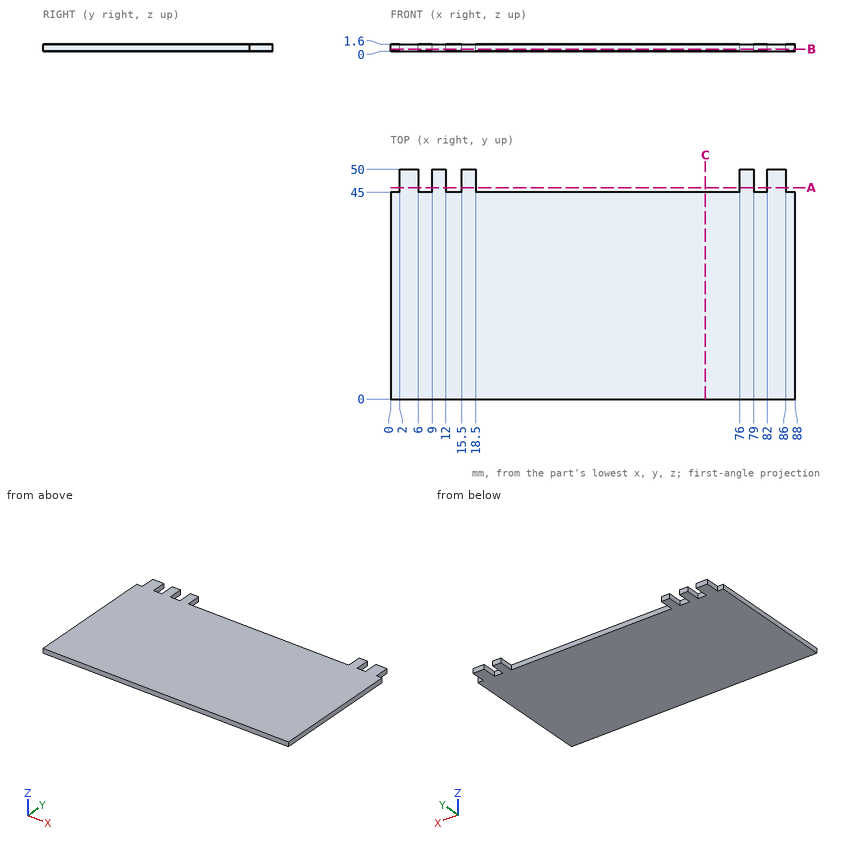
Source: three-view drawing plus pictorial views. Frame: mm from the lowest corner of the part. Give positions to 0.01 mm unless a question says otherwise; leave off trailing zeros. Write each loop counter-clockwise with the first axis right and the second up, starting at its lowest first coordinate (ties: lowest second). Pieces come first, ordered by that corner, then holes. Notation, with made-up numbers: M -5,68 L 1,68 A14 cw 1,72 Z; hole C -36,-17.5 d3. An arc over 180 degrees is marked long. Use one line per item in the form item = value.
1. Ray query, L1, parallel to X at y = 47.5, z = 1.15; L2, parallel to Y at x = 36, z = 1.35. Return the intervals inside material, ascending.
Outcome:
L1 = 2 to 6, 9 to 12, 15.5 to 18.5, 76 to 79, 82 to 86
L2 = 0 to 45
2. First-contact query: P1, Ø0.8, axis at x = 45.5, z = 1, coming from the +Y side; P2, Ø0.8, axis at y = 47.5, z = 1, coming from the -X side; P3, Ø0.5, axis at y = 47.5, z = 1, coming from the +X side. Flat tips, straight axial feed; report the tip coordinate or a pass-through.
Outcome:
P1 = 45
P2 = 2
P3 = 86
3. Cut plane B-B on z = 0.5. Return loops of the section in (x, y).
Outcome:
outline = M 0,0 L 88,0 L 88,45 L 86,45 L 86,50 L 82,50 L 82,45 L 79,45 L 79,50 L 76,50 L 76,45 L 18.5,45 L 18.5,50 L 15.5,50 L 15.5,45 L 12,45 L 12,50 L 9,50 L 9,45 L 6,45 L 6,50 L 2,50 L 2,45 L 0,45 Z
4. Cut plane A-A on y = 46. Return loops of the section in (x, z), and give its area (3 significant figures).
Outcome:
outline = M 2,0 L 6,0 L 6,1.6 L 2,1.6 Z; M 9,0 L 12,0 L 12,1.6 L 9,1.6 Z; M 15.5,0 L 18.5,0 L 18.5,1.6 L 15.5,1.6 Z; M 76,0 L 79,0 L 79,1.6 L 76,1.6 Z; M 82,0 L 86,0 L 86,1.6 L 82,1.6 Z
area = 27.2 mm²
5. Cut plane C-C on x = 68.5. Return loops of the section in (y, z), and give its area (3 significant figures).
Outcome:
outline = M 0,0 L 45,0 L 45,1.6 L 0,1.6 Z
area = 72.0 mm²
